Geometry check sheet. Reference: the model listing, model coordinates, mm. A direction names the side the tool comes from. Give positions to 0.01 mm unless a question says otherwise; leave off trailing zeros. Order: outer loops, then holes, each group sorted by start corner. A loop starts at its lowest first (then second) coordinate and runs counter-clockwise, first axis right, second up. Notation, with made-up numbers: M 55.25,-36.75 L 96.25,-36.75 A35 cw 96.25,1.25 Z; hole C -30.75,3 d8. An arc over 180 degrees is marked long. Answer as CSV lines item,"result". Start each with the question number.
```python
from build123d import *

# Parameters (mm, degrees)
F0_W     = 157.48
F0_H     = 76.2
F1_DEPTH = 6.35
F2_W     = 157.48
F2_H     = 12.7
F3_DEPTH = 31.75
F4_W     = 157.48
F4_H     = 6.35
F5_DEPTH = 6.35
F7_D     = 12.7
F8_W     = 3.302
F8_H     = 63.5
F9_DEPTH = 25.4
F11_D    = 12.7


with BuildPart() as f1:
    # F0 (on Front) → F1 (new body)
    with BuildSketch(Plane.XZ):
        with Locations((-16.753665, -12.914129)):
            Rectangle(F0_W, F0_H)
    extrude(amount=F1_DEPTH)

    # F2 (on face) → F3 (join)
    with BuildSketch(Plane.XZ.offset(6.35)):
        with Locations((-16.753665, -44.664129)):
            Rectangle(F2_W, F2_H)
    extrude(amount=F3_DEPTH)

    # F4 (on face) → F5 (join)
    with BuildSketch(Plane.XY.offset(-38.314129)):
        with Locations((-16.753665, -34.925)):
            Rectangle(F4_W, F4_H)
    extrude(amount=F5_DEPTH)

    # F7 (through all)
    with Locations(Plane.XY.offset(-38.314129)):
        with Locations((-16.753665, -19.05)):
            Hole(F7_D / 2)

    # F8 (on face) → F9 (join)
    with BuildSketch(Plane.XZ.offset(6.35)):
        with Locations((-93.842665, -6.564129)):
            Rectangle(F8_W, F8_H)
        with Locations((60.335335, -6.564129)):
            Rectangle(F8_W, F8_H)
    extrude(amount=F9_DEPTH)

    # F11 (through all)
    with Locations(Plane.YZ.offset(61.986335)):
        with Locations((-17.52157, -8.528198)):
            Hole(F11_D / 2)


solid = f1.part
```
Item 1: Access from +Z, -Z, +X, -X, +Y, -Y to the whole of each face (thin tool, end or side, straight path). Record for faces 4 (the face through (-92.192, -25, -7)), 5 (the face through (-22.62, -21.48, -44.75)), 6 (the face through (60, -31.75, -3)).
Item 2: Scan lines: line 1 along X through (y, z) = (-9, 16.5); line 2 along Y through (x, z) = (-20.5, -34.5); line 3 along Z through (x, y) = (-6, -9.5). Record each from-to range of solid material in increasing order.
Item 3: Draft check along Y on faces 1 (the face through (-93.87, -12.84, -4.24)), 2 (the face through (-17, -4, 25.186)), 3 (the face through (-18, 0, -12)). Enter one of: pulls with the +Y half, pulls with the -Y half, needs draft (parallel to the pull), parting line crosses it, or undercut.
Item 4: Section check C-C on z = 20.5. Record the boundary of the cut face in (x, y), then the cut area to 3 significant figures.
Item 5: Depth check by flat-ended pin: pin 1 Ø8 at (x, z) = (36.5, 7) entering from -Y; pin 2 Ø3 at (x, y) = (-0.5, -35.5) entering from +Z; pin 3 Ø1 at (x, y) = (10, -11) entering from +Z; pin 4 Ø20.5 at (y, z) = (-16, -6.5) entering from +X. Enter the tip coordinate at first touch or a pass-through.
Item 6: Section check A-A on y = -19.05. Record the boundary of the cut face in (x, z), then the cut area to 3 significant figures.
Item 7: Section check D-D on z = -11.5. Record the boundary of the cut face in (x, y), then the cut area to 3 significant figures.
Item 8: Section check B-B on x = -28.5. Record the boundary of the cut face in (y, z), then the cut area to 3 significant figures.
Numbers:
1,face 4,"+Z"
1,face 5,"+Z, -Z"
1,face 6,"+Z, +X, -X, -Y"
2,line 1,"-95.49 to -92.19, 58.68 to 61.99"
2,line 2,"-38.1 to -31.75, -6.35 to 0"
2,line 3,"-51.01 to -38.31"
3,face 1,"undercut"
3,face 2,"needs draft"
3,face 3,"pulls with the +Y half"
4,outline,"M -95.49,-31.75 L -92.19,-31.75 L -92.19,-6.35 L 58.68,-6.35 L 58.68,-31.75 L 61.99,-31.75 L 61.99,0 L -95.49,0 Z"
4,area,"1,170 mm2"
5,pin 1,"y = -6.35"
5,pin 2,"z = -31.96"
5,pin 3,"z = -38.31"
5,pin 4,"x = 61.99"
6,outline,"M -95.49,-51.01 L -23.1,-51.01 L -23.1,-38.31 L -92.19,-38.31 L -92.19,-14.69 L -95.49,-14.69 Z; M -95.49,-2.36 L -92.19,-2.36 L -92.19,25.19 L -95.49,25.19 Z; M -10.4,-51.01 L 61.99,-51.01 L 61.99,-14.69 L 58.68,-14.69 L 58.68,-38.31 L -10.4,-38.31 Z; M 58.68,-2.36 L 61.99,-2.36 L 61.99,25.19 L 58.68,25.19 Z"
6,area,"2,180 mm2"
7,outline,"M -95.49,-31.75 L -92.19,-31.75 L -92.19,-23.13 L -95.49,-23.13 Z; M -95.49,-11.91 L -92.19,-11.91 L -92.19,-6.35 L 58.68,-6.35 L 58.68,-11.91 L 61.99,-11.91 L 61.99,0 L -95.49,0 Z; M 58.68,-31.75 L 61.99,-31.75 L 61.99,-23.13 L 58.68,-23.13 Z"
7,area,"1,090 mm2"
8,outline,"M -38.1,-51.01 L 0,-51.01 L 0,25.19 L -6.35,25.19 L -6.35,-38.31 L -31.75,-38.31 L -31.75,-31.96 L -38.1,-31.96 Z"
8,area,"927 mm2"
